Study the drawing (mm; zero at the part's minimum x, y, z) and answer. A direction names the side the tool comes from. Give positions to 0.01 mm unless a question says otherwise; leave off trailing zeros. Write each loop counter-clockwise with the first axis right and the second up, starting at its lowest first coordinate (ties: lowest second). Pieces come first, ordered by that corner, then holes. Notation, with made-up numbers: (27.5, 23) - (80.5, 23) arc R11 ccw to (80.5, 31) - close; hole circle Ø2 at (19, 24). An arc over 180 degrees is marked (long way). Return JSON: item names as keys, results as strings.
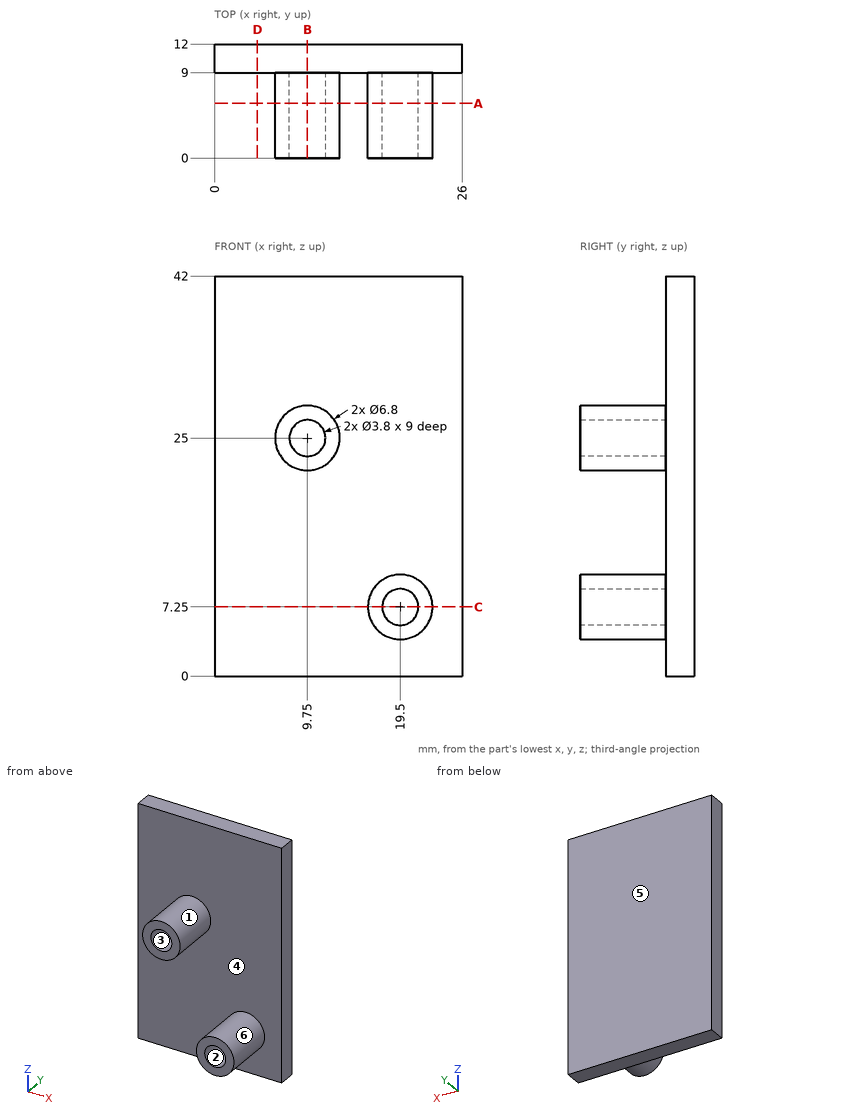
Item 1: A cutting plane is placed at C-C on z = 7.25. Determine the outline of the cut face in (x, y).
Answer below:
{"outline": "(0, 9) - (16.1, 9) - (16.1, 0) - (17.6, 0) - (17.6, 9) - (21.4, 9) - (21.4, 0) - (22.9, 0) - (22.9, 9) - (26, 9) - (26, 12) - (0, 12) - close"}
Item 2: A cutting plane is placed at A-A on y = 5.75. Determine the outline of the cut face in (x, z).
Answer below:
{"outline": "circle Ø6.8 at (9.75, 25); circle Ø6.8 at (19.5, 7.25); hole circle Ø3.8 at (9.75, 25); hole circle Ø3.8 at (19.5, 7.25)"}
Item 3: Consider L1, parallel to X at y = 3, z = 7.25; L2, parallel to X at y = 2.5, z = 25; L3, parallel to Y at x = 13, z = 3.5. Determine where each line is inside the solid, lowest interval first.
Answer below:
{"L1": "x = 16.1 to 17.6, 21.4 to 22.9", "L2": "x = 6.35 to 7.85, 11.65 to 13.15", "L3": "y = 9 to 12"}
Item 4: For the marked faces 5 and 6, determine the directions among +Z, -Z, +X, -X, +Y, -Y from which every point of the face is accessible in a straight line to the end or side of a thin tool.
Answer below:
{"face 5": "+Z, -Z, +X, -X, +Y", "face 6": "-Y"}
Item 5: A cutting plane is placed at B-B on x = 9.75. Determine the outline of the cut face in (y, z), then the cut area to 3 significant figures.
Answer below:
{"outline": "(0, 21.6) - (9, 21.6) - (9, 0) - (12, 0) - (12, 42) - (9, 42) - (9, 28.4) - (0, 28.4) - (0, 26.9) - (9, 26.9) - (9, 23.1) - (0, 23.1) - close", "area": "153 mm²"}
Item 6: The mould has two halves that part along Z. Classify the marked faces 1, 2, 3 and 4: +Z half, -Z half, draft (parallel to the pull), parting line (faces both ways), or undercut.
Answer below:
{"face 1": "parting line", "face 2": "undercut", "face 3": "undercut", "face 4": "draft"}
Item 7: A cutting plane is placed at D-D on x = 4.5. Determine the outline of the cut face in (y, z), then the cut area to 3 significant figures.
Answer below:
{"outline": "(9, 0) - (12, 0) - (12, 42) - (9, 42) - close", "area": "126 mm²"}
Item 8: Flat-ended cylindrical pins translate along their axes: P1, Ø8, axis at x = 13, z = 16, coming from the -Y side; P2, Ø4, axis at y = 5, z = 9, coming from the -X side; P3, Ø5, axis at x = 13, y = 3, coming from the -Z side. Find the tip coordinate at first contact, or state that the pin passes through.
Answer below:
{"P1": "stops at y = 9", "P2": "stops at x = 16.1", "P3": "stops at z = 21.68"}
